Autodesk Inventor part; units mm, degrees
ref_plane "Work Plane2" through (-4.0424, 1.7685, 44.45) normal (0, 0, 1) x (1, 0, 0)
ref_plane "YZ Plane" through (0, 0, 0) normal (1, 0, 0) x (0, 1, 0)
ref_plane "XZ Plane" through (0, 0, 0) normal (0, 1, 0) x (-1, 0, 0)
sketch "Sketch1" plane through (0, 0, 0) normal (0, 0, 1) x (1, 0, 0)
  arc A0 (-4.0424, -42.6815) -> (40.4076, 1.7685) centre (-4.0424, 1.7685) ccw
  line L0 (-4.0424, 1.7685) -> (40.4076, 1.7685)
  line L1 (-4.0424, 1.7685) -> (-4.0424, -42.6815)
  dimension "d0" = 88.9
revolve "Revolution1" add sketch "Sketch1" angle 360 about axis through (-4.0424, 1.7685, 0) along (0, -1, 0)
ref_plane "Work Plane2" through (-4.0424, 1.7685, 44.45) normal (0, 0, 1) x (1, 0, 0)
sketch "Sketch3" plane through (-4.0424, 1.7685, 44.45) normal (0, 0, 1) x (1, 0, 0)
  line L0 (-27.3232, -41.3412) -> (29.0699, -41.3412)
surface extrude "ExtrusionSrf2" sketch "Sketch3" against normal blind 127 shown no curves L0
split body "Split2" result one side removed by surface "ExtrusionSrf2" removed pieces at (7.0948, -40.569, -3.8851)
shell "Shell2" thickness 3.175 removed faces 1 at (-16.0293, 1.7685, -8.709)
properties part number "ORB-bottom"
For this review, take the finished solid that the model builds, in its own axes (mm). Coordinates: 2 decimals unless noted, no trailing zeros. Write each loop counter-clockwise with the first axis right and the second up, starting at its lowest first coordinate (ties: lowest second). Pieces come first, ordered by that corner, then holes.
(1) Add section D-D on x = -30. Give the boundary of the cut face in (y, z).
(2) The part is to be moulded in two halves that separate along Z. For faces 1 (the face through (-4, -36.398, 0)), 2 (the face through (-4, -39.573, 0)), say which applies: +Z half, -Z half, draft (parallel to the pull), parting line (faces both ways), or undercut.
(3) For pin 1 Ø12 at (x, y) = (-30, -35) entering from -Z; pin 2 Ø8 at (y, z) = (-5.5, -22.5) entering from +X; pin 3 Ø8 at (x, z) = (25.5, -15.5) entering from +Y, all flat-tipped, find the tip position at first contact; note any pin that passes through.
(4) Add section C-C on y = -26. Give the boundary of the cut face in (x, z), then the cut area to 3 significant figures.
(5) Add section B-B on x = -8. Give the boundary of the cut face in (y, z).
(6) Add section A-A on z = 7. Give the boundary of the cut face in (x, y).
(7) Wall thickness on probe 1 along X at (y, z) = (-0.5, 17.5) (3 decimals); probe 2 along X at (y, z) = (-7, 3); probe 3 along Z at (x, y) = (-11.5, -35): over which ranges is each line inside the solid? List them lowest first.
Answer sheet:
1. outline: (1.77, -36.08) - (1.77, -32.09) arc R32.09 cw to (1.77, 32.09) - (1.77, 36.08) arc R36.08 ccw to start
2. face 1: undercut
2. face 2: draft
3. pin 1: stops at z = -21.31
3. pin 2: stops at x = 35.83
3. pin 3: stops at y = -15.77
4. outline: circle Ø69.42 at (-4.04, 0); hole circle Ø61.07 at (-4.04, 0)
4. area: 855 mm2
5. outline: (-39.57, -15.84) arc R44.27 ccw to (1.77, -44.27) - (1.77, -41.08) arc R41.08 cw to (-36.4, -15.21) - (-36.4, 15.21) arc R41.08 cw to (1.77, 41.08) - (1.77, 44.27) arc R44.27 ccw to (-39.57, 15.84) - close
6. outline: (-47.94, 1.77) arc R43.9 ccw to (-18.8, -39.57) - (10.71, -39.57) arc R43.9 ccw to (39.85, 1.77) - (36.63, 1.77) arc R40.68 cw to (10.03, -36.4) - (-18.11, -36.4) arc R40.68 cw to (-44.72, 1.77) - close
7. probe 1: x = -44.84 to -41.355, 33.27 to 36.755
7. probe 2: x = -47.52 to -44.26, 36.18 to 39.43
7. probe 3: z = -23.84 to -17.21, 17.21 to 23.84
